Input: dimensioned drawing with shaded views. Units: mm. Origin: part minimum x, y, z. A direction names the side the tool comes from. Coordinates: 2 decimals unless noted, no trailing zeros. Order: outer loops, then holes, each group sorted by start corner. A loop starts at its lowest first (then second) coordinate and runs counter-clockwise, first axis right, second up. Notation, with made-up numbers: (-25.5, -1.5) -> (-3.5, -1.5) arc R17 ccw to (-3.5, 27.5) -> close; hole circle Ø5 at (51.5, 7.5). An arc over 180 degrees is marked (long way). Write item = value, one per line. Start each with the question number.
Item 1: Section query A-A (z = 23). Output: boundary loops of the cut face in (x, y), then the cut area to 3 significant figures.
Item 2: Section query D-D (y = 7.5). Output: boundary loops of the cut face in (x, z).
Item 3: Contact query for flat-ended pins moving along their axis: pin 1 (3 mm diameter, centred on x = 43, z = 4.5, fed in from +Y); pin 2 (1.5 mm diameter, centred on x = 17.5, z = 10, fed in from -Y); pin 3 (0.6 mm diameter, centred on y = 1, z = 10.5, fed in from -X); pin 4 (3 mm diameter, centred on x = 32, z = 23, fed in from -Y). Output: stop coordinate, or through.
Item 4: Ray query, line 1 along Z through (x, y) = (32, 9.75); line 2 along Z through (x, y) = (6, 0.7); line 3 along X through (y, z) = (3.25, 5.25). Return the intervals inside material, ascending. Write a range as [from, to].
Item 5: Section query C-C (y = 3.5). Output: boundary loops of the cut face in (x, z).
Item 6: Mould query, pull axis Z, two halves, no side actions, for the marked faces 3, 4 and 5. Classes: released by +Z, released by -Z, zero draft, split by the parting line, or undercut.
Item 7: Section query B-B (x = 27.5). Output: boundary loops of the cut face in (y, z), then the cut area to 3 significant figures.
Item 8: Set-up query: the marked faces 1 and 2. Return all of +Z, -Z, +X, -X, +Y, -Y with unobstructed straight access to the full face (end or side cutting, diameter ignored); none if empty.
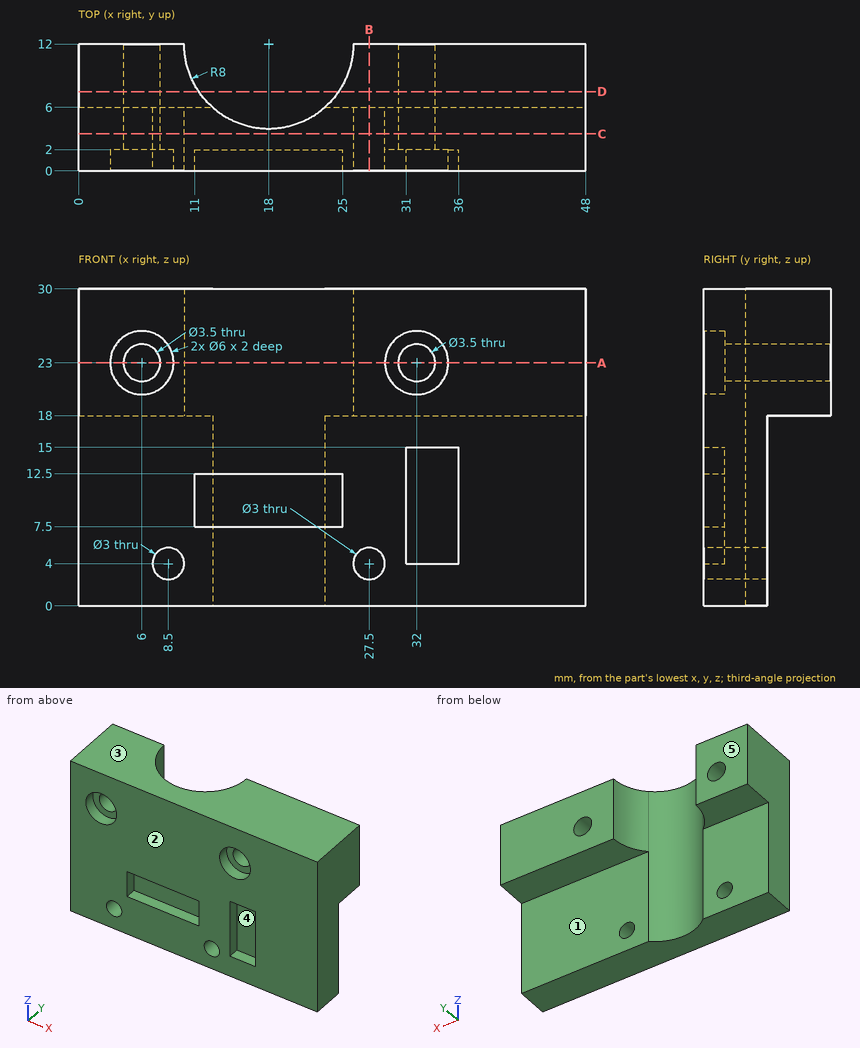
Computed:
q1.outline = (0, 0) -> (3, 0) -> (3, 2) -> (4.25, 2) -> (4.25, 12) -> (0, 12) -> close; (7.75, 2) -> (9, 2) -> (9, 0) -> (29, 0) -> (29, 2) -> (30.25, 2) -> (30.25, 12) -> (26, 12) arc R8 cw to (10, 12) -> (7.75, 12) -> close; (33.75, 2) -> (35, 2) -> (35, 0) -> (48, 0) -> (48, 12) -> (33.75, 12) -> close
q1.area = 381 mm^2
q2.outline = (0, 18) -> (11.39, 18) -> (11.39, 30) -> (0, 30) -> close; (24.61, 18) -> (48, 18) -> (48, 30) -> (24.61, 30) -> close; hole circle Ø3.5 at (6, 23); hole circle Ø3.5 at (32, 23)
q3.pin_1 = 6
q3.pin_2 = 2
q3.pin_3 = 0
q3.pin_4 = through
q4.line_1 = [18, 21.25], [24.75, 30]
q4.line_2 = [0, 20], [26, 30]
q4.line_3 = [0, 7.67], [9.33, 26.67], [28.33, 48]
q5.outline = (0, 0) -> (48, 0) -> (48, 30) -> (0, 30) -> close; hole circle Ø3.5 at (6, 23); hole circle Ø3 at (8.5, 4); hole circle Ø3 at (27.5, 4); hole circle Ø3.5 at (32, 23)
q6.face_3 = released by +Z
q6.face_4 = undercut
q6.face_5 = zero draft
q7.outline = (0, 0) -> (6, 0) -> (6, 2.5) -> (0, 2.5) -> close; (0, 5.5) -> (6, 5.5) -> (6, 18) -> (12, 18) -> (12, 30) -> (0, 30) -> close
q7.area = 234 mm^2
q8.face_1 = -Z, +X, -X, +Y
q8.face_2 = +Z, -Z, +X, -X, -Y
